Study the drawing (mm; zero at the part's minimum x, y, z) and answer. A direction names the side the tool comes from. Round coordinates to 2 decimals unless told otherwise and drop trailing zeros. Write each loop counter-clockwise with the first axis right and the second up, starting at its lowest first coordinate (ties: lowest second). Pieces come first, ordered by that corner, then holes.
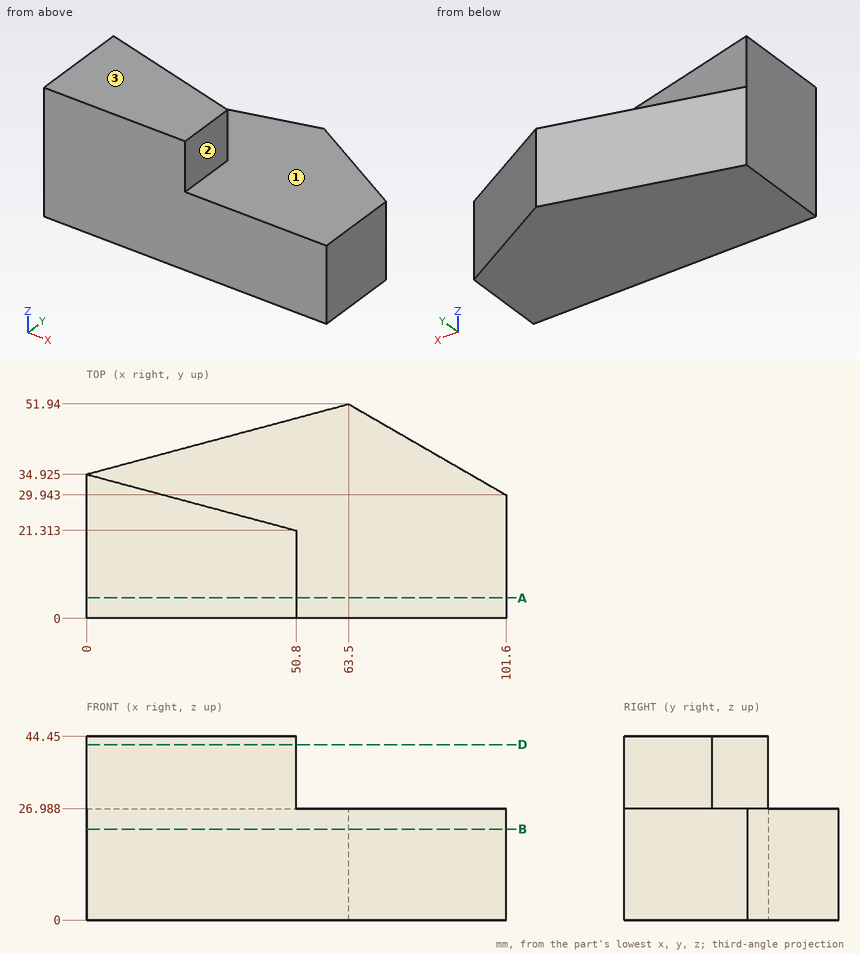
Q1. Find section D-D (z = 42.5). Determine the outline of the cut face in (x, y) (1 decimal).
Q2. Find section B-B (z = 22). Determine the outline of the cut face in (x, y) (1 decimal).
Q3. A tool of negligible diameter and unlimited length cuts with its end or side. For the marked faces 1, 2 and 3, from which of +Z, -Z, +X, -X, +Y, -Y can it reach the whole face along a straight path? Write none if from no direction.
Q4. Find the intervals of material crossed by L1, parallel to X at y = 8.5, z = 33.5; L2, parallel to Z at x = 27.5, y = 39; L3, parallel to Y at x = 86, z = 5, in increasing order.
Q5. Find section A-A (y = 5). Determine the outline of the cut face in (x, z), plus the area to 3 significant figures.
Q6. Given pin 1 (1.5 mm diameter, centred on x = 82, z = 23, fed in from +Y); pin 2 (14 mm diameter, centred on y = 8.5, z = 36, fed in from +X); pin 3 (4 mm diameter, centred on x = 74, z = 23.5, fed in from +Y), each flat-ended and moving along its own axis, determine where each tip first touches the part or whether it passes through.
Report:
1. outline: (0, 0) - (50.8, 0) - (50.8, 21.3) - (0, 34.9) - close
2. outline: (0, 0) - (101.6, 0) - (101.6, 29.9) - (63.5, 51.9) - (0, 34.9) - close
3. face 1: +Z, +X, +Y
3. face 2: +Z, +X, +Y, -Y
3. face 3: +Z, +X, -X, +Y, -Y
4. L1: x = 0 to 50.8
4. L2: z = 0 to 26.99
4. L3: y = 0 to 38.95
5. outline: (0, 0) - (101.6, 0) - (101.6, 26.99) - (50.8, 26.99) - (50.8, 44.45) - (0, 44.45) - close
5. area: 3,630 mm2
6. pin 1: stops at y = 41.69
6. pin 2: stops at x = 50.8
6. pin 3: stops at y = 47.03
